Verification items for the finished model (mm, model axes). Face numbers are marked on the shaded views. A direction names the side the tool comes from. Round coordinates to 2 decimals unless told otherwise and drop trailing zeros. Order: outer loops, then holes, each group sorted by start corner. A loop starts at its lowest first (then second) coordinate and runs counter-clockwise, first axis right, second up. Notation, with made-up numbers: (-5, 64) -> (26, 64) arc R32 cw to (26, 92) -> close; hole circle Ø3 at (-8, 29.25). An arc over 180 degrees is marked (long way). Put each result on its own line as item: value.
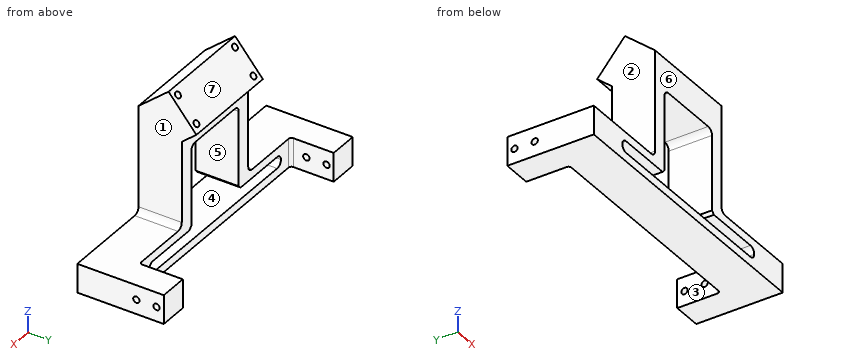
from build123d import *

# Parameters (mm, degrees)
BOSS_EXTRUDE1_DEPTH = 12.7
SKETCH2_R           = 1.397
CUT_EXTRUDE1_DEPTH  = 133.569206561
FILLET1_R           = 1.27
BOSS_EXTRUDE2_DEPTH = 22.225
CUT_EXTRUDE3_DEPTH  = 97.775414884
FILLET3_R           = 2.54
CHAMFER1_SIZE       = 1.27
SKETCH7_R           = 1.397
CUT_EXTRUDE4_DEPTH  = 6.35


with BuildPart() as part:
    # Sketch1 → Boss-Extrude1 (new body)
    with BuildSketch(Plane.XY):
        Polygon((63.1698, 0), (-63.1698, 0), (-63.1698, 38.1), (-50.4698, 38.1), (-50.4698, 19.05), (50.4698, 19.05), (50.4698, 38.1), (63.1698, 38.1), align=None)
    extrude(amount=BOSS_EXTRUDE1_DEPTH)

    # Sketch2 → Cut-Extrude1 (cut, through all)
    with BuildSketch(Plane.ZY.offset(63.1698)):
        with Locations((6.35, 34.925)):
            Circle(SKETCH2_R)
        with Locations((6.35, 26.035)):
            Circle(SKETCH2_R)
    extrude(amount=-CUT_EXTRUDE1_DEPTH, mode=Mode.SUBTRACT)

    # Fillet1
    fillet1_edges = [part.edges().sort_by_distance(p)[0] for p in [
        (-50.4698, 19.05, 6.35),
        (50.4698, 19.05, 6.35),
    ]]
    fillet(fillet1_edges, radius=FILLET1_R)

    # Sketch3 → Boss-Extrude2 (add, symmetric)
    with BuildSketch(Plane(origin=(0, 0, 0), x_dir=(0, 0, -1), z_dir=(1, 0, 0))):
        Polygon((-12.7, 19.05), (-12.7, 0), (-59.683160888, 0), (-70.796573321, 13.244449193), (-56.203426679, 25.489553157), (-50.8, 19.05), align=None)
    extrude(amount=BOSS_EXTRUDE2_DEPTH, both=True)

    # Sketch6 → Cut-Extrude3 (cut, through all)
    with BuildSketch(Plane(origin=(0, 19.05, 0), x_dir=(1, 0, 0), z_dir=(0, 1, 0))):
        Polygon((44.1198, -3.81), (-44.1198, -3.81), (-44.1198, -8.89), (-15.875, -8.89), (-15.875, -45.72), (15.875, -45.72), (15.875, -8.89), (44.1198, -8.89), align=None)
    extrude(amount=-CUT_EXTRUDE3_DEPTH, mode=Mode.SUBTRACT)

    # Fillet3
    fillet3_edges = [part.edges().sort_by_distance(p)[0] for p in [
        (44.1198, 9.525, 8.89),
        (44.1198, 9.525, 3.81),
        (15.875, 9.525, 45.72),
        (-15.875, 9.525, 45.72),
        (-44.1198, 9.525, 8.89),
        (-44.1198, 9.525, 3.81),
        (22.225, 9.525, 12.7),
        (-22.225, 9.525, 12.7),
    ]]
    fillet(fillet3_edges, radius=FILLET3_R - 0.0001)  # a hair under: the kernel refuses the full size

    # Chamfer1
    chamfer1_edges = [part.edges().sort_by_distance(p)[0] for p in [
        (15.875, 9.525, 8.89),
        (-15.875, 9.525, 8.89),
    ]]
    chamfer(chamfer1_edges, length=CHAMFER1_SIZE)

    # Sketch7 → Cut-Extrude4 (cut, symmetric)
    with BuildSketch(Plane(origin=(0, 42.632668976, 35.773056814), x_dir=(1, 0, 0), z_dir=(0, 0.7660444431189747, 0.6427876096865435))):
        with Locations(Location((-19.05, -29.844953746, 0), (0, 0, 270))):
            Circle(SKETCH7_R)
        with Locations(Location((-19.05, -42.544953746, 0), (0, 0, 90))):
            Circle(SKETCH7_R)
        with Locations(Location((19.05, -42.544953746, 0), (0, 0, 270))):
            Circle(SKETCH7_R)
        with Locations(Location((19.05, -29.844953746, 0), (0, 0, 90))):
            Circle(SKETCH7_R)
    extrude(amount=CUT_EXTRUDE4_DEPTH, both=True, mode=Mode.SUBTRACT)


solid = part.part
Item 1: Release check for a two-part mould opening along Z. For the marked faces 4, 5, 6 and 7 record: +Z half, -Z half, draft (parallel to the pull), parting line (faces both ways), or undercut.
Check sheet entries:
face 4: undercut
face 5: undercut
face 6: draft
face 7: +Z half
Item 2: Gauge pin test, flat ends, axial feed: pin 1 Ø1.5 at (y, z) = (15, 53.5) entering from -X (3 decimals); pin 2 Ø15 at (y, z) = (10.5, 33.5) entering from +X (3 decimals); pin 3 Ø12 at (x, y) = (-26.5, 33) entering from -Z; pin 4 Ø1.5 at (x, y) = (18.5, 25) entering from +Z. Record the tip position at first contact, or that the pin passes through.
Check sheet entries:
pin 1: stops at x = -22.225
pin 2: stops at x = 22.225
pin 3: passes through
pin 4: stops at z = 57.68
Item 3: Section check A-A on x = -30.5. Record the boundary of the cut face in (y, z), then the cut area to 3 significant figures.
Check sheet entries:
outline: (0, 0) -> (19.05, 0) -> (19.05, 3.81) -> (0, 3.81) -> close; (0, 8.89) -> (19.05, 8.89) -> (19.05, 12.7) -> (0, 12.7) -> close
area: 145 mm^2
Item 4: Section check D-D on x = 6. Record the boundary of the cut face in (y, z), then the cut area to 3 significant figures.
Check sheet entries:
outline: (0, 0) -> (19.05, 0) -> (19.05, 3.81) -> (0, 3.81) -> close; (0, 45.72) -> (19.05, 45.72) -> (19.05, 50.8) -> (25.49, 56.2) -> (13.24, 70.8) -> (0, 59.68) -> close
area: 499 mm^2
Item 5: Tool access check on the marked faces 1, 2 and 3. Record the directions out of +Z, -Z, +X, -X, +Y, -Y that give a thin tool (end or side, any length) a straight path to the whole face; none if there is none.
Check sheet entries:
face 1: +Z, +X, +Y, -Y
face 2: +Z, -X, +Y, -Y
face 3: +Z, -Z, +Y
Item 6: Material ranges on L1, parallel to Y at x = -53.25, z = 6.35; L2, parallel to Z at x = 41, y = 15; L3, parallel to Y at x = 55, z = 6, recorded low to high. Write a range as [from, to].
Check sheet entries:
L1: y = [0, 24.64], [27.43, 33.53], [36.32, 38.1]
L2: z = [0, 3.81], [8.89, 12.7]
L3: y = [0, 24.68], [27.39, 33.57], [36.28, 38.1]
Item 7: Section check B-B on z = 31. Record the boundary of the cut face in (x, y) (3 decimals), then the cut area to 3 significant figures.
Check sheet entries:
outline: (-22.225, 0) -> (-15.875, 0) -> (-15.875, 19.05) -> (-22.225, 19.05) -> close; (15.875, 0) -> (22.225, 0) -> (22.225, 19.05) -> (15.875, 19.05) -> close
area: 242 mm^2
